Design review of the part built by this model. Coordinates are the model's own, in mm. Coordinates: 2 decimals unless noted, no trailing zeros. Loops run counter-clockwise (first coordinate to the right, second up) from the corner with the lowest first, then second, coordinate; pieces in that order, holes last. Notation, with made-up numbers: (-13, -0.5) -> (8, -0.5) arc R3 cw to (8, 4.5) -> close; hole circle Ø5 at (26.5, 76). An arc over 180 degrees is marked (long way). Use a Markdown table: item, result. Add a question column.
Q1. Take a section at A-A on z = -21. Write out the cut boundary in (x, y).
Q2. Draft analysis for pull direction X (two halves, no side actions). For faces 1 (the face through (120.759, -9.515, -1.498)), 2 (the face through (119.92, -8.234, -1.498)), 3 (the face through (3, -1, 107)), state which applies: pulls with the +X half, pulls with the -X half, needs draft (parallel to the pull), parting line crosses it, or undercut.
Q3. For probe 1 along X at (y, z) = (-5.75, 57); probe 2 along Y at (x, z) = (117, 62); probe 3 along Y at (x, z) = (77, 70), list the stretches that pass through material, from the lowest coordinate up.
Q4. Clearance check with flat-ended pins moving along their axes: pin 1 Ø3 at (x, z) = (-21, -58.5) entering from -Y; pin 2 Ø2 at (y, z) = (-9.5, 6.5) entering from -X; pin 3 Ø1.5 at (y, z) = (-7, -12) entering from -X. State where each tip first meets the part, or that it passes through.
Q5. Take a section at B-B on x = 57.5. Write out the cut boundary in (y, z).
from build123d import *

# Parameters (mm, degrees)
SKETCH_1_W             = 234
SKETCH_1_H             = 214
SM_BASE_FLANGE_1_DEPTH = 1.5
OTHER_START            = -107
OTHER_1_DEPTH          = 214
FILLET_3_R             = 1.5


# Read off the part's stored shape, not the designer's step: Каемка1
# Sheet-metal steps are written as plain solids
with BuildPart() as part:
    # Sketch 1 → Базовая кромка1 (new body)
    with BuildSketch(Plane.XZ.offset(1.5)):
        Rectangle(SKETCH_1_W, SKETCH_1_H)
    extrude(amount=-SM_BASE_FLANGE_1_DEPTH)

    # Other 1 outline → Other 1 (add)
    with BuildSketch(Plane.XY.offset(OTHER_START)):
        with BuildLine():
            Line((113, -5.5), (111.5, -5.5))
            ThreePointArc((111.5, -5.5), (120.889087297, -9.389087297), (117, 0))
            Line((117, 0), (117, -1.5))
            ThreePointArc((117, -1.5), (119.828427125, -8.328427125), (113, -5.5))
        make_face()
    extrude(amount=OTHER_1_DEPTH)

    # Скругление3
    # the kernel refuses this fillet: 1.5 mm, written as the material it takes off along each edge
    with BuildSketch(Plane(origin=(-117, 0, -110.75), x_dir=(0, -1, 0), z_dir=(0, 0, 1))) as fillet_3_piece_1:
        with BuildLine():
            CenterArc((FILLET_3_R, FILLET_3_R), FILLET_3_R, 180, 90)
            Line((0, FILLET_3_R), (0, 0))
            Line((0, 0), (FILLET_3_R, 0))
        make_face()
    extrude(amount=221.5, mode=Mode.SUBTRACT)
    with BuildSketch(Plane(origin=(-117, -1.5, -110.75), x_dir=(0, 1, 0), z_dir=(0, 0, 1))) as fillet_3_piece_2:
        with BuildLine():
            CenterArc((FILLET_3_R, -FILLET_3_R), FILLET_3_R, 90, 90)
            Line((0, -FILLET_3_R), (0, 0))
            Line((0, 0), (FILLET_3_R, 0))
        make_face()
    extrude(amount=221.5, mode=Mode.SUBTRACT)
    with BuildSketch(Plane(origin=(-117, -5.25, -107), x_dir=(0, 0, 1), z_dir=(0, 1, 0)), Plane(origin=(-117, -5.25, 107), x_dir=(1, 0, 0), z_dir=(0, 1, 0))) as fillet_3_piece_3:
        with BuildLine():
            CenterArc((FILLET_3_R, FILLET_3_R), FILLET_3_R, 180, 90)
            Line((0, FILLET_3_R), (0, 0))
            Line((0, 0), (FILLET_3_R, 0))
        make_face()
    extrude(amount=9, mode=Mode.SUBTRACT)


solid = part.part
Answer list:
| question | item | result |
|---|---|---|
| 1 | outline | (-116.8, -0.75) arc R1.5 ccw to (-115.5, -1.5) -> (117, -1.5) arc R4 cw (long way) to (113, -5.5) -> (111.5, -5.5) arc R5.5 ccw (long way) to (117, 0) -> (-115.5, 0) arc R1.5 ccw to start |
| 2 | face 1 | parting line crosses it |
| 2 | face 2 | undercut |
| 2 | face 3 | needs draft |
| 3 | probe 1 | 111.51 to 113.01, 120.99 to 122.49 |
| 3 | probe 2 | -11 to -9.5, -1.5 to 0 |
| 3 | probe 3 | -1.5 to 0 |
| 4 | pin 1 | y = -1.5 |
| 4 | pin 2 | x = 112.39 |
| 4 | pin 3 | x = 111.55 |
| 5 | outline | (-1.5, -107) -> (0, -107) -> (0, 107) -> (-1.5, 107) -> close |
